For this review, take the finished solid that the model builds, in its own axes (mm). A direction names the side the tool comes from. Round coordinates to 2 decimals unless told otherwise and drop trailing zeros. Write each loop counter-clockwise with the first axis right and the second up, starting at its lowest first coordinate (ties: lowest second). Pieces come first, ordered by that corner, then holes. Notation, with made-up numbers: (7.25, 22.5) -> (46.25, 22.5) arc R22 ccw to (46.25, 41.5) -> close; hole circle Ø6 at (-0.75, 13). An arc over 180 degrees is marked (long way). Answer as CSV lines item,"result". Start each with the question number.
Item 1: Take a section at A-A on z = -47. Give the boundary of the cut face in (x, y).
Item 2: Machinability: for faces 1 (the flat face through (-10, 4, -4)), 2 (the flat face through (5, 4, -4)), 3 (the flat face through (9, 2, -62)), 4 (the flat face through (0, 0, -51)), 5 (the cylindrical face through (6.51, 4.74, -3.45)), which of the approach directions +Z, -Z, +X, -X, +Y, -Y give a long, thin tool a straight path to every point of the face, cutting with its end or side? Answer none if there is none.
Item 3: Take a section at D-D on x = 7.75. Give the boundary of the cut face in (y, z), then the cut area to 3 significant figures.
Item 4: Take a section at C-C on x = 0. Give the boundary of the cut face in (y, z), then the cut area to 4 significant figures.
Item 5: Wall thickness on probe 1 along X at (y, z) = (1.75, -74); probe 2 along Y at (x, z) = (0, -3.5); probe 3 along Z at (x, y) = (6, 4): over which ranges is each line inside the solid? List them lowest first. Write a range as from..to.
Item 6: Take a section at B-B on y = 2. Give the boundary of the cut face in (x, z).
Item 7: Mouldability with a two-part tool opening along Z and no side actions: class faces 6 (the cylindrical face through (-11.15, 1.52, -96.99)), 7 (the flat face through (-9, 2, -62)), 8 (the flat face through (-14, 1, -44)) as +Z half, -Z half, draft (parallel to the pull), parting line (faces both ways), or undercut.
Item 8: For pin 1 Ø12 at (x, z) = (6.5, -62.5) entering from +Y; pin 2 Ø2 at (y, z) = (4.5, -4.5) entering from -X; pin 3 Ø1.5 at (x, y) = (6.5, 4.5) entering from -Z; pin 4 Ø1.5 at (x, y) = (-11, 2.5) entering from +Z, all flat-tipped, find the tip position at first contact; note any pin that passes through.
```python
from build123d import *

# Parameters (mm, degrees)
CROQUIS1_W              = 28
CROQUIS1_H              = 100
SALIENTE_EXTRUIR1_DEPTH = 3
CROQUIS2_W              = 28
CROQUIS2_H              = 7
SALIENTE_EXTRUIR2_DEPTH = 5
CORTAR_EXTRUIR2_REACH   = 102
CROQUIS3_R              = 1.25
CORTAR_EXTRUIR3_START   = -7
CORTAR_EXTRUIR3_DEPTH   = 7
CORTAR_EXTRUIR4_DEPTH   = 10
REDONDEO1_R             = 10


with BuildPart() as part:
    # Croquis1 → Saliente-Extruir1 (new body)
    with BuildSketch(Plane(origin=(0, 0, 0), x_dir=(1, 0, 0), z_dir=(0, 1, 0))):
        with Locations((0, 50)):
            Rectangle(CROQUIS1_W, CROQUIS1_H)
    extrude(amount=SALIENTE_EXTRUIR1_DEPTH)

    # Croquis2 → Saliente-Extruir2 (add)
    with BuildSketch(Plane(origin=(0, 3, 0), x_dir=(1, 0, 0), z_dir=(0, 1, 0))):
        with Locations((0, 3.5)):
            Rectangle(CROQUIS2_W, CROQUIS2_H)
    extrude(amount=SALIENTE_EXTRUIR2_DEPTH)

    # Croquis3 → Cortar-Extruir2 (cut, up to next)
    with BuildSketch(Plane.XY, mode=Mode.PRIVATE) as cortar_extruir2_sk1:
        with Locations((-7.5, 5.5)):
            Circle(CROQUIS3_R)
    cortar_extruir2_tool1 = extrude(cortar_extruir2_sk1.sketch, amount=-CORTAR_EXTRUIR2_REACH, mode=Mode.PRIVATE) & part.part
    add(cortar_extruir2_tool1.solids().sort_by_distance((-7.5, 5.5, 0))[0], mode=Mode.SUBTRACT)
    # Croquis3 → Cortar-Extruir2 (cut, up to next)
    with BuildSketch(Plane.XY, mode=Mode.PRIVATE) as cortar_extruir2_sk2:
        with Locations((0, 5.5)):
            Circle(CROQUIS3_R)
    cortar_extruir2_tool2 = extrude(cortar_extruir2_sk2.sketch, amount=-CORTAR_EXTRUIR2_REACH, mode=Mode.PRIVATE) & part.part
    add(cortar_extruir2_tool2.solids().sort_by_distance((0, 5.5, 0))[0], mode=Mode.SUBTRACT)
    # Croquis3 → Cortar-Extruir2 (cut, up to next)
    with BuildSketch(Plane.XY, mode=Mode.PRIVATE) as cortar_extruir2_sk3:
        with Locations((7.5, 5.5)):
            Circle(CROQUIS3_R)
    cortar_extruir2_tool3 = extrude(cortar_extruir2_sk3.sketch, amount=-CORTAR_EXTRUIR2_REACH, mode=Mode.PRIVATE) & part.part
    add(cortar_extruir2_tool3.solids().sort_by_distance((7.5, 5.5, 0))[0], mode=Mode.SUBTRACT)

    # Croquis4 → Cortar-Extruir3 (cut)
    with BuildSketch(Plane.XY.offset(CORTAR_EXTRUIR3_START)):
        with BuildLine():
            Line((-10, 3), (-14, 3))
            Line((-14, 3), (-14, 8))
            Line((-14, 8), (-14, 10.200483226))
            Line((-14, 10.200483226), (14, 10.200483226))
            Line((14, 10.200483226), (14, 8))
            Line((14, 8), (14, 3))
            Line((14, 3), (10, 3))
            Line((10, 3), (10, 5.5))
            ThreePointArc((10, 5.5), (7.5, 8), (5, 5.5))
            Line((5, 5.5), (5, 3))
            Line((5, 3), (2.5, 3))
            Line((2.5, 3), (2.5, 5.5))
            ThreePointArc((2.5, 5.5), (0, 8), (-2.5, 5.5))
            Line((-2.5, 5.5), (-2.5, 3))
            Line((-2.5, 3), (-5, 3))
            Line((-5, 3), (-5, 5.5))
            ThreePointArc((-5, 5.5), (-7.5, 8), (-10, 5.5))
            Line((-10, 5.5), (-10, 3))
        make_face()
    extrude(amount=CORTAR_EXTRUIR3_DEPTH, mode=Mode.SUBTRACT)

    # Croquis5 → Cortar-Extruir4 (cut)
    with BuildSketch(Plane(origin=(0, 3, 0), x_dir=(1, 0, 0), z_dir=(0, 1, 0))):
        with BuildLine():
            Line((-9, 32), (-9, 93.208471881))
            ThreePointArc((-9, 93.208471881), (-7.5, 94.708471881), (-6, 93.208471881))
            Line((-6, 93.208471881), (-6, 32))
            ThreePointArc((-6, 32), (-7.5, 30.5), (-9, 32))
        make_face()
        with BuildLine():
            Line((9, 32), (9, 93.208471881))
            ThreePointArc((9, 93.208471881), (7.5, 94.708471881), (6, 93.208471881))
            Line((6, 93.208471881), (6, 32))
            ThreePointArc((6, 32), (7.5, 30.5), (9, 32))
        make_face()
    extrude(amount=-CORTAR_EXTRUIR4_DEPTH, mode=Mode.SUBTRACT)

    # Redondeo1
    redondeo1_edges = [part.edges().sort_by_distance(p)[0] for p in [
        (-14, 1.5, -100),
        (14, 1.5, -100),
    ]]
    fillet(redondeo1_edges, radius=REDONDEO1_R)


solid = part.part
```
Output values:
1,outline,"(-14, 0) -> (-9, 0) -> (-9, 3) -> (-14, 3) -> close; (-6, 0) -> (6, 0) -> (6, 3) -> (-6, 3) -> close; (9, 0) -> (14, 0) -> (14, 3) -> (9, 3) -> close"
2,face 1,"+Z, -Z, -X, +Y"
2,face 2,"+Z, -Z, +Y"
2,face 3,"+Y, -Y"
2,face 4,"+Z, -Z, +X, -X, -Y"
2,face 5,"+Z, -Z"
3,outline,"(0, -99.27) -> (3, -99.27) -> (3, -94.69) -> (0, -94.69) -> close; (0, -30.52) -> (3, -30.52) -> (3, -7) -> (4.28, -7) -> (4.28, 0) -> (0, 0) -> close; (6.72, -7) -> (7.99, -7) -> (7.99, 0) -> (6.72, 0) -> close"
3,area,"123 mm^2"
4,outline,"(0, -100) -> (3, -100) -> (3, -7) -> (4.25, -7) -> (4.25, 0) -> (0, 0) -> close; (6.75, -7) -> (8, -7) -> (8, 0) -> (6.75, 0) -> close"
4,area,"317.5 mm^2"
5,probe 1,"x = -14..-9, -6..6, 9..14"
5,probe 2,"y = 0..4.25, 6.75..8"
5,probe 3,"z = -7..0"
6,outline,"(-14, -90) arc R10 ccw to (-4, -100) -> (4, -100) arc R10 ccw to (14, -90) -> (14, 0) -> (-14, 0) -> close; hole (-9, -93.21) arc R1.5 ccw to (-6, -93.21) -> (-6, -32) arc R1.5 ccw to (-9, -32) -> close; hole (6, -93.21) arc R1.5 ccw to (9, -93.21) -> (9, -32) arc R1.5 ccw to (6, -32) -> close"
7,face 6,"-Z half"
7,face 7,"undercut"
7,face 8,"draft"
8,pin 1,"stops at y = 3"
8,pin 2,"stops at x = -10"
8,pin 3,"stops at z = -7"
8,pin 4,"stops at z = 0"
